```python
from build123d import *

# Parameters (mm, degrees)
F1_DEPTH      = 1
F1_DEPTH_BACK = 1
F2_R          = 0.5


with BuildPart() as f1:
    # F0 (on Top) → F1 (new body, two sides)
    with BuildSketch(Plane.XY) as f1_sk:
        Polygon((7, 9.248056), (7, 48.79661), (4, 48.79661), (4, 9.248056), (4.890339, 9.248056), (4.890339, 17.506754), (6.190339, 17.506754), (6.190339, 9.248056), align=None)
    extrude(amount=F1_DEPTH)
    extrude(f1_sk.sketch, amount=-F1_DEPTH_BACK)

    # F2
    f2_edges = [f1.edges().sort_by_distance(p)[0] for p in [
        (4, 29.022333, 1),
        (7, 29.022333, 1),
    ]]
    fillet(f2_edges, radius=F2_R)


solid = f1.part
```
Here's how the part is built. I have some questions about the finished solid (model axes, mm). A direction names the side the tool comes from. Round coordinates to 2 decimals unless told otherwise and drop trailing zeros. Loops run counter-clockwise (first coordinate to the right, second up) from the corner with the lowest first, then second, coordinate; pieces in that order, holes last.
1. For faces 4 (the face through (6.6, 9.248, 0)), 5 (the face through (6.19, 13, 0)), which set-ups out of +Z, -Z, +X, -X, +Y, -Y let a thin tool reach every point of the face, with its end or its side?
Answers:
face 4: +Z, -Z, +X, -X, -Y
face 5: +Z, -Z, -Y
2. If I drill on probe 1 along X at (y, z) = (15.5, -0.55); probe 2 along Y at (x, z) = (5.3, -0.75); probe 3 along X at (y, z) = (11.5, 0.9), over which ranges is the centre line in solid material (lowest first)?
Answers:
probe 1: x = 4 to 4.89, 6.19 to 7
probe 2: y = 17.51 to 48.8
probe 3: x = 4.2 to 4.89, 6.19 to 6.8
3. Suppose I cut it at A-A, the plane z = -0.5. Please give me the cut outline in (x, y).
Answers:
outline: (4, 9.25) - (4.89, 9.25) - (4.89, 17.51) - (6.19, 17.51) - (6.19, 9.25) - (7, 9.25) - (7, 48.8) - (4, 48.8) - close
4. Thinking about a two-plate mould opening in X: for faces 1 (the face through (6, 17.507, 0)), 2 (the face through (5, 34, 1)), 3 (the face through (7, 29, 0)), which applies, released by +X, released by -X, zero draft, split by the parting line, or undercut?
Answers:
face 1: undercut
face 2: zero draft
face 3: released by +X
5. Suppose I cut it at B-B, the plane y = 37. Please give me the cut outline in (x, z), and give its area (3 significant figures).
Answers:
outline: (4, -1) - (7, -1) - (7, 0.5) arc R0.5 ccw to (6.5, 1) - (4.5, 1) arc R0.5 ccw to (4, 0.5) - close
area: 5.89 mm2
6. Suppose I cut it at C-C, the plane x = 5.6. Please give me the cut outline in (y, z).
Answers:
outline: (17.51, -1) - (48.8, -1) - (48.8, 1) - (17.51, 1) - close
